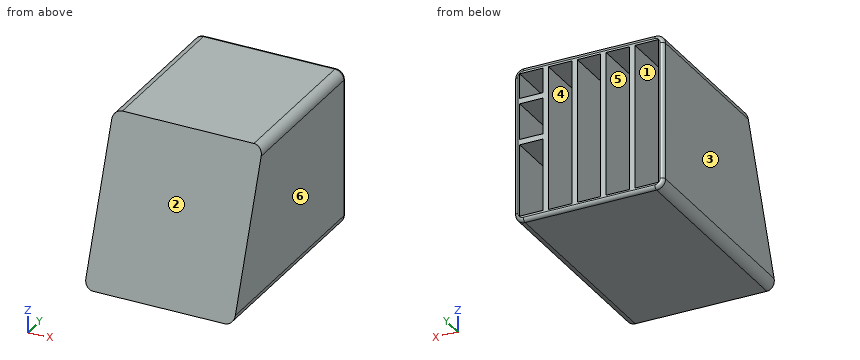
Autodesk Fusion 360 part; units mm, degrees
sketch "Sketch1" plane through (0, 0, 0) normal (0, 1, 0) x (1, 0, 0)
  line L0 (41.5, 43) -> (-41.5, 43)
  line L1 (-41.5, 43) -> (-41.5, -43)
  line L2 (-41.5, -43) -> (41.5, -43)
  line L3 (41.5, -43) -> (41.5, 43)
  line L4 (41.5, 43) -> (-41.5, -43) construction
  line L5 (-41.5, 43) -> (41.5, -43) construction
  line L6 (-38.5, -39.8916) -> (-25.5, -39.8916)
  line L7 (-25.5, -39.8916) -> (-25.5, 40.1084)
  line L8 (-25.5, 40.1084) -> (-38.5, 40.1084)
  line L9 (-38.5, 40.1084) -> (-38.5, -39.8916)
  line L10 (-22.5, 40.1084) -> (-22.5, -39.8916)
  line L11 (-9.5, 40.1084) -> (-22.5, 40.1084)
  line L12 (-9.5, -39.8916) -> (-9.5, 40.1084)
  line L13 (-22.5, -39.8916) -> (-9.5, -39.8916)
  line L14 (-6.5, 40.1084) -> (-6.5, -39.8916)
  line L15 (6.5, 40.1084) -> (-6.5, 40.1084)
  line L16 (6.5, -39.8916) -> (6.5, 40.1084)
  line L17 (-6.5, -39.8916) -> (6.5, -39.8916)
  line L18 (9.5, 40.1084) -> (9.5, -39.8916)
  line L19 (22.5, 40.1084) -> (9.5, 40.1084)
  line L20 (22.5, -39.8916) -> (22.5, 40.1084)
  line L21 (9.5, -39.8916) -> (22.5, -39.8916)
  line L22 (38.5, 39.8916) -> (25.5, 39.8916)
  line L23 (25.5, 39.8916) -> (25.5, -0.1084)
  line L24 (25.5, -0.1084) -> (38.5, -0.1084)
  line L25 (38.5, -0.1084) -> (38.5, 39.8916)
  line L26 (38.5, -3.1084) -> (25.5, -3.1084)
  line L27 (25.5, -3.1084) -> (25.5, -23.1084)
  line L28 (25.5, -23.1084) -> (38.5, -23.1084)
  line L29 (38.5, -23.1084) -> (38.5, -3.1084)
  line L30 (38.5, -39.8916) -> (25.5, -39.8916)
  line L31 (25.5, -39.8916) -> (25.5, -26.1084)
  line L32 (25.5, -26.1084) -> (38.5, -26.1084)
  line L33 (38.5, -26.1084) -> (38.5, -39.8916)
  dimension "d1" = 83
  dimension "d2" = 86
  dimension "d3" = 80
  dimension "d4" = 13
  dimension "d5" = 3
  dimension "d8" = 48
  dimension "d9" = 0
  dimension "d10" = 3
  dimension "d11" = 40
  dimension "d12" = 3
  dimension "d13" = 3
  dimension "d14" = 20
  dimension "d17" = 13
  dimension "d18" = 3
  dimension "d19" = 3
extrude "Extrude1" add sketch "Sketch1" along normal blind 70 contours L0 L1 L2 L3 | L6 L7 L8 L9 | L10 L11 L12 L13 | L14 L15 L16 L17 | L18 L19 L20 L21 | L22 L23 L24 L25 | L26 L27 L28 L29 | L30 L31 L32 L33
extrude "Extrude2" add sketch "Sketch1" along normal blind 50 from surface at 70
sketch "Sketch2" plane through (41.5, 0, 0) normal (1, 0, 0) x (0, 0, -1)
  line L0 (-43, 0) -> (43, 0)
  line L1 (43, 0) -> (43, 120)
  line L2 (43, 120) -> (-43, 120)
  line L3 (-43, 120) -> (-43, 0)
  line L4 (-43, 31.3014) -> (43, 0)
  dimension "d29" = 20
extrude "Extrude4" cut sketch "Sketch2" against normal up to surface (83 mm away) contours L0 L3 L4
fillet "Fillet2" radius 5 4 edges at (41.5, 75.6507, 43) (-41.5, 75.6507, 43) (41.5, 60, -43) (-41.5, 60, -43)
fillet "Fillet3" radius 2 8 edges at (40.0355, 120, 41.5355) (41.5, 120, 0) (40.0355, 120, -41.5355) (0, 120, -43) (-40.0355, 120, -41.5355) (-41.5, 120, 0) (-40.0355, 120, 41.5355) (0, 120, 43)
equation "d1 = ( ( 13 + 3 ) * 5 ) * 1 mm + 3 mm"
equation "d2 = 80 mm + 6 mm"
equation "d8 = ( 16 * 3 ) * 1 mm"
Verification items for the finished model (mm, model axes). Face numbers are marked on the shaded views. A direction names the side the tool comes from. Give positions to 0.01 mm unless a question says otherwise; leave off trailing zeros. Order: outer loops, then holes, each group sorted by start corner. A loop starts at its lowest first (then second) coordinate and runs counter-clockwise, first axis right, second up. Notation, with made-up numbers: M 58,55 L 80,55 A29 ccw 80,81 Z; hole C -9.75,23 d9. An arc over 180 degrees is marked long. Use one line per item in the form item = value. Start each with the question number.
Q1. Section check B-B (z = 34). Enter the section's corners in (x, y).
Q2. Section check A-A (x = -11.5). Enter the section's corners in (y, z).
Q3. Scan lines: line 1 along X through (y, z) = (101.5, 24.5); line 2 along X through (y, z) = (71.5, -10.5); line 3 along Z through (x, y) = (33, 87.5). Record each from-to range of solid material in increasing order. Write a range as [from, to].
Q4. Section check D-D (x = 32). Enter the section's corners in (y, z), then the cut area to 3 significant figures.
Q5. Go/stop test with flat-tipped pins: pin 1 Ø4 at (x, z) = (-32, -11.5) entering from +Y; pin 2 Ø12 at (x, z) = (-5.5, -24) entering from -Y; pin 3 Ø12 at (x, z) = (-5, -2) entering from -Y. Record where each tip stops, or that it passes through.
Q6. Section check C-C (y = 112.5). Count the separate pieces of the cut face and the enclosed holes in it, then the cut area to 3 significant figures.
Q7. Mould release check, pull along X, two halves, no side actions. Record for the marked faces 3, 4, 5 and 6: +X half, -X half, draft (parallel to the pull), parting line (faces both ways), or undercut.
Q8. Access from +Z, -Z, +X, -X, +Y, -Y to the whole of each face (thin tool, end or side, straight path). Record for the marked faces 1 and 2.
Evaluation:
q1.outline = M -41.5,28.03 L 41.5,28.03 L 41.5,118 A2 ccw 39.5,120 L 38.5,120 L 38.5,70 L 25.5,70 L 25.5,120 L 22.5,120 L 22.5,70 L 9.5,70 L 9.5,120 L 6.5,120 L 6.5,70 L -6.5,70 L -6.5,120 L -9.5,120 L -9.5,70 L -22.5,70 L -22.5,120 L -25.5,120 L -25.5,70 L -38.5,70 L -38.5,120 L -39.5,120 A2 ccw -41.5,118 Z
q2.outline = M 0,-43 L 118,-43 A2 ccw 120,-41 L 120,-40.11 L 70,-40.11 L 70,39.89 L 120,39.89 L 120,41 A2 ccw 118,43 L 31.3,43 Z
q3.line_1 = [-41.5, -38.5], [-25.5, -22.5], [-9.5, -6.5], [6.5, 9.5], [22.5, 41.5]
q3.line_2 = [-41.5, -38.5], [-25.5, -22.5], [-9.5, -6.5], [6.5, 9.5], [22.5, 25.5], [38.5, 41.5]
q3.line_3 = [-43, -39.89], [0.11, 3.11], [23.11, 26.11], [39.89, 43]
q4.outline = M 0,-43 L 118,-43 A2 ccw 120,-41 L 120,-39.89 L 70,-39.89 L 70,0.11 L 120,0.11 L 120,3.11 L 70,3.11 L 70,23.11 L 120,23.11 L 120,26.11 L 70,26.11 L 70,39.89 L 120,39.89 L 120,41 A2 ccw 118,43 L 31.3,43 Z
q4.area = 5,280 mm2
q5.pin_1 = 70
q5.pin_2 = 4.73
q5.pin_3 = 12.74
q6.separate_pieces = 1
q6.enclosed_holes = 7
q6.area = 2,000 mm2
q7.face_3 = -X half
q7.face_4 = undercut
q7.face_5 = undercut
q7.face_6 = +X half
q8.face_1 = +Y
q8.face_2 = +Z, +X, -X, -Y
